Work out the finished part from the listing and answer in its coordinate system (mm). Face numbers are marked on the shaded views. Coordinates: 2 decimals unless noted, no trailing zeros. Loops run counter-clockwise (first coordinate to the right, second up) from the corner with the lowest first, then second, coordinate; pieces in that order, holes last. Notation, with made-up numbers: (21, -29) -> (39, -29) arc R17 cw to (39, -12) -> close; hole circle Ø11 at (13.25, 16). An arc over 180 degrees is marked (long way). Answer as CSV lines item,"result".
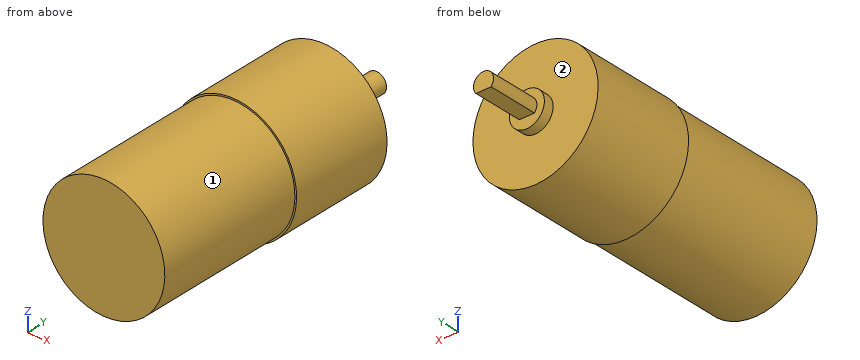
```python
from build123d import *

# Parameters (mm, degrees)
SKETCH1_W           = 12.075
SKETCH1_H           = 30
SKETCH2_W           = 12.4
SKETCH2_H           = 20.86
SKETCH3_R           = 3.48
BOSS_EXTRUDE1_DEPTH = 2
BOSS_EXTRUDE2_DEPTH = 10


with BuildPart() as part:
    # Sketch1 → Revolve1 (revolve)
    with BuildSketch(Plane(origin=(0, 0, 0), x_dir=(0, 0, -1), z_dir=(1, 0, 0))):
        with Locations((6.0375, -16.859504132)):
            Rectangle(SKETCH1_W, SKETCH1_H)
    revolve(axis=Axis((0, 44.256198347, 0), (0, -1, 0)))

    # Sketch2 → Revolve2 (revolve)
    with BuildSketch(Plane(origin=(0, 0, 0), x_dir=(0, 0, -1), z_dir=(1, 0, 0))):
        with Locations((6.2, 8.570495868)):
            Rectangle(SKETCH2_W, SKETCH2_H)
    revolve(axis=Axis((0, -1.859504132, 0), (0, 1, 0)))

    # Sketch3 → Boss-Extrude1 (add)
    with BuildSketch(Plane(origin=(0, 19.000495868, 0), x_dir=(1, 0, 0), z_dir=(0, 1, 0))):
        Circle(SKETCH3_R)
    extrude(amount=BOSS_EXTRUDE1_DEPTH)

    # Sketch4 → Boss-Extrude2 (add)
    with BuildSketch(Plane(origin=(0, 21.000495868, 0), x_dir=(1, 0, 0), z_dir=(0, 1, 0))):
        with BuildLine():
            Line((-1.5, 1.305560373), (1.5, 1.305560373))
            ThreePointArc((1.5, 1.305560373), (0, -1.988589421), (-1.5, 1.305560373))
        make_face()
    extrude(amount=BOSS_EXTRUDE2_DEPTH)


solid = part.part
```
(1) A cutting plane is placed at C-C, the plane y = 6. Write down the section's boundary in (x, z), and give its area (3 significant figures).
Computed values:
outline,"circle Ø24.8 at (0, 0)"
area,"483 mm2"
(2) Flat-ended cylindrical pins translate along their axes: pin 1 Ø3 at (x, z) = (9.5, -8.5) entering from +Y; pin 2 Ø6 at (y, z) = (-20, 0) entering from +X (3 decimals); pin 3 Ø6 at (x, y) = (6, 7) entering from -Z. Find the tip coordinate at first contact, or state that the pin passes through.
Computed values:
pin 1,"y = 19"
pin 2,"x = 12.075"
pin 3,"z = -12.03"
(3) Consider line 1 along Y through (x, z) = (-8.5, -5); line 2 along Y through (x, z) = (3.25, 1); line 3 along X through (y, z) = (4.5, -7). Determine where each line is inside the solid, lowest interval first.
Computed values:
line 1,"-31.86 to 19"
line 2,"-31.86 to 21"
line 3,"-10.24 to 10.24"
(4) A cutting plane is placed at B-B, the plane z = 6.25. Write down the section's boundary in (x, y).
Computed values:
outline,"(-10.71, -1.86) -> (-10.33, -1.86) -> (-10.33, -31.86) -> (10.33, -31.86) -> (10.33, -1.86) -> (10.71, -1.86) -> (10.71, 19) -> (-10.71, 19) -> close"
(5) For a pull along Z with two mould halves and no side action, classify the marked faces 1 and 2 as pulls with the +Z half, pulls with the -Z half, needs draft (parallel to the pull), parting line crosses it, or undercut.
Computed values:
face 1,"parting line crosses it"
face 2,"needs draft"
(6) A cutting plane is placed at D-D, the plane x = 6. Write down the section's boundary in (y, z).
Computed values:
outline,"(-31.86, -10.48) -> (-1.86, -10.48) -> (-1.86, -10.85) -> (19, -10.85) -> (19, 10.85) -> (-1.86, 10.85) -> (-1.86, 10.48) -> (-31.86, 10.48) -> close"
